from build123d import *

# Parameters (mm, degrees)
CROQUIS1_R                    = 135
BRIDA_BASE1_DEPTH             = 4
CROQUIS6_R                    = 1.65
CROQUIS6_R_2                  = 6.05
CROQUIS6_R_3                  = 12.25
CROQUIS6_R_4                  = 7.75
CORTAR_EXTRUIR1_DEPTH         = 10
TALADRO_DE_MARGEN_PARA_1_41_D = 6.7564
CROQUIS11_R                   = 10.05
CORTAR_EXTRUIR3_DEPTH         = 10
TALADRO_DE_MARGEN_PARA_M51_D  = 5.2
TALADRO_DE_MARGEN_PARA_M52_D  = 5.2
CROQUIS16_R                   = 5
CORTAR_EXTRUIR4_DEPTH         = 191.960728947


# Sheet-metal steps are written as plain solids
with BuildPart() as part:
    # Croquis1 → Brida base1 (new body)
    with BuildSketch(Plane(origin=(0, 0, 0), x_dir=(1, 0, 0), z_dir=(0, 1, 0))):
        with Locations(Location((0, 0, 0), (0, 0, 270))):
            Circle(CROQUIS1_R)
    extrude(amount=-BRIDA_BASE1_DEPTH)

    # Croquis6 → Cortar-Extruir1 (cut)
    with BuildSketch(Plane(origin=(0, 0, 0), x_dir=(1, 0, 0), z_dir=(0, 1, 0))):
        with Locations(Location((43.718012531, 54.678167639, 0), (0, 0, 270))):
            Circle(CROQUIS6_R)
        with Locations(Location((47.72970773, 69.650017947, 0), (0, 0, 270))):
            Circle(CROQUIS6_R)
        with Locations(Location((63.639610307, 63.639610307, 0), (0, 0, 270))):
            Circle(CROQUIS6_R_2)
        with Locations(Location((63.639610307, -63.639610307, 0), (0, 0, 270))):
            Circle(CROQUIS6_R_3)
        with Locations(Location((-63.639610307, 63.639610307, 0), (0, 0, 270))):
            Circle(CROQUIS6_R_4)
        with Locations(Location((62.701558038, 73.661713146, 0), (0, 0, 270))):
            Circle(CROQUIS6_R)
        with Locations(Location((73.661713146, 62.701558038, 0), (0, 0, 270))):
            Circle(CROQUIS6_R)
        with Locations(Location((69.650017947, 47.72970773, 0), (0, 0, 270))):
            Circle(CROQUIS6_R)
        with Locations(Location((54.678167639, 43.718012531, 0), (0, 0, 270))):
            Circle(CROQUIS6_R)
    extrude(amount=-CORTAR_EXTRUIR1_DEPTH, mode=Mode.SUBTRACT)

    # Taladro de margen para 1/41 (through all)
    with Locations(Plane(origin=(0, 0, 0), x_dir=(1, 0, 0), z_dir=(0, 1, 0))):
        with Locations((100, 0), (60, 0), (0, -100), (0, -60), (-100, 0), (-60, 0), (0, 100), (0, 60), (0, 0)):
            Hole(TALADRO_DE_MARGEN_PARA_1_41_D / 2)

    # Croquis11 → Cortar-Extruir3 (cut)
    with BuildSketch(Plane(origin=(0, 0, 0), x_dir=(1, 0, 0), z_dir=(0, 1, 0))):
        with Locations(Location((0, 0, 0), (0, 0, 270))):
            Circle(CROQUIS11_R)
    extrude(amount=-CORTAR_EXTRUIR3_DEPTH, mode=Mode.SUBTRACT)

    # Taladro de margen para M51 (through all)
    with Locations(Plane(origin=(0, 0, 0), x_dir=(1, 0, 0), z_dir=(0, 1, 0))):
        with Locations((17, 17), (-17, 17), (-17, -17), (17, -17)):
            Hole(TALADRO_DE_MARGEN_PARA_M51_D / 2)

    # Taladro de margen para M52 (through all)
    with Locations(Plane(origin=(0, 0, 0), x_dir=(1, 0, 0), z_dir=(0, 1, 0))):
        with Locations((-33.510619649, -66.744638365), (-66.744638365, -99.97865708), (-99.97865708, -66.744638365), (-66.744638365, -33.510619649), (-66.744638365, -66.744638365)):
            Hole(TALADRO_DE_MARGEN_PARA_M52_D / 2)

    # Croquis16 → Cortar-Extruir4 (cut, through all)
    with BuildSketch(Plane(origin=(0, 0, 0), x_dir=(1, 0, 0), z_dir=(0, 1, 0))):
        with Locations(Location((-66.744638365, -66.744638365, 0), (0, 0, 270))):
            Circle(CROQUIS16_R)
    extrude(amount=-CORTAR_EXTRUIR4_DEPTH, mode=Mode.SUBTRACT)


solid = part.part
Could you check a few things on this model? Use its own coordinates, in mm. Give positions to 0.01 mm unless a question says otherwise; leave off trailing zeros. Loops run counter-clockwise (first coordinate to the right, second up) from the corner with the lowest first, then second, coordinate; pieces in that order, holes last. Notation, with made-up numbers: M 77.25,28.5 L 109.25,28.5 A9 cw 109.25,34.5 Z; hole C 72,88 d8. An arc over 180 degrees is marked long. Answer as a JSON object with one key per item and string values.
Q1. Suppose I cut it at C-C, the plane y = -2.8. State how many separate pieces and enclosed holes the cut face has, plus the area to 3 significant figures.
Values found:
{"separate pieces": "1", "enclosed holes": "27", "area": "55,600 mm²"}
Q2. Suppose I cut it at B-B, the plane x = 0. List the corners of the cut face in (y, z) for me.
Values found:
{"outline": "M -4,-135 L 0,-135 L 0,-103.38 L -4,-103.38 Z; M -4,-96.62 L 0,-96.62 L 0,-63.38 L -4,-63.38 Z; M -4,-56.62 L 0,-56.62 L 0,-10.05 L -4,-10.05 Z; M -4,10.05 L 0,10.05 L 0,56.62 L -4,56.62 Z; M -4,63.38 L 0,63.38 L 0,96.62 L -4,96.62 Z; M -4,103.38 L 0,103.38 L 0,135 L -4,135 Z"}
Q3. Suppose I cut it at D-D, the plane x = 32.5. List the corners of the cut face in (y, z) for me, plus the area to 3 significant figures.
Values found:
{"outline": "M -4,-131.03 L 0,-131.03 L 0,131.03 L -4,131.03 Z", "area": "1,050 mm²"}
Q4. Suppose I cut it at A-A, the plane z = 0. List the corners of the cut face in (x, y) for me, plus the area to 4 significant figures.
Values found:
{"outline": "M -135,-4 L -103.38,-4 L -103.38,0 L -135,0 Z; M -96.62,-4 L -63.38,-4 L -63.38,0 L -96.62,0 Z; M -56.62,-4 L -10.05,-4 L -10.05,0 L -56.62,0 Z; M 10.05,-4 L 56.62,-4 L 56.62,0 L 10.05,0 Z; M 63.38,-4 L 96.62,-4 L 96.62,0 L 63.38,0 Z; M 103.38,-4 L 135,-4 L 135,0 L 103.38,0 Z", "area": "891.5 mm²"}
Q5. If I drill on probe 1 along Z at (x, y) = (-1, -3.15); probe 2 along Z at (x, y) = (59.5, -0.4); probe 3 along X at (y, z) = (-1.75, -62.5), over which ranges is the centre line in solid material (lowest first)? Write a range as [from, to].
Values found:
{"probe 1": "z = [-135, -103.23], [-96.77, -63.23], [-56.77, -10], [10, 56.77], [63.23, 96.77], [103.23, 135]", "probe 2": "z = [-121.18, -68.05], [-59.23, -3.34], [3.34, 52.11], [75.17, 121.18]", "probe 3": "x = [-119.66, -71.31], [-55.97, -2.27], [2.27, 57.7], [69.58, 72.02], [75.3, 119.66]"}
Q6. For P1, Ø1, axis at y = -1, z = -47, coming from the -X side; P2, Ø1.5, axis at x = -9, y = -1, coming from the -Z side, each with a flat end and sliding along its axis, tell me the tip position at first contact or that it passes through.
Values found:
{"P1": "stops at x = -126.74", "P2": "stops at z = -134.75"}
Q7. If we mould it in two halves opening along Z, with no side actions, what happens to faces 1 (the cylindrical face through (-119.77, -1.97, 62.29)), 2 (the flat face through (-28, -4, -2)), 3 (the cylindrical face through (0.44, -1.97, -10.04))? For each: pulls with the +Z half, pulls with the -Z half, needs draft (parallel to the pull), parting line crosses it, or undercut.
Values found:
{"face 1": "parting line crosses it", "face 2": "needs draft", "face 3": "undercut"}
